CAD build for the part. Positions are in the model's coordinates, mm. Coordinates: 2 decimals unless noted, no trailing zeros. Loops run counter-clockwise (first coordinate to the right, second up) from the corner with the lowest first, then second, coordinate; pieces in that order, holes last.
1) Saw through at A-A, the plane x = 7. Write the cut outline in (y, z).
2) Pin check, flat tips, straight feed: pin 1 Ø8 at (x, y) = (11.5, -7) entering from +Z; pin 2 Ø5 at (x, z) = (2.5, 24.5) entering from +Y; pin 3 Ø4.5 at (x, z) = (7.5, 0) entering from -Y. Stop position of each tip, or through.
3) Saw through at B-B, the plane y = 0. Write the cut outline in (x, z), and give its area (3 significant figures).
4) Wall check: line 1 along X through (y, z) = (79, 0); line 2 along Z through (x, y) = (6, -70); line 3 along Y through (x, z) = (9.5, 43). Give the ranges that are in metal, low to high.
5) Two-plate mould, pull along Z, no slides. Class faces 1 (the flat face through (0, 17, 75)), 2 (the cylindrical face through (6, 81, 2)): +Z half, -Z half, draft (parallel to the pull), parting line (faces both ways), or undercut.
```python
from build123d import *

# Parameters (mm, degrees)
SKETCH1_W                      = 14
SKETCH1_H                      = 2
CUT_EXTRUDE1_REACH             = 123.723
SKETCH1_3_R                    = 2.5
CUT_EXTRUDE1_DIRECTION_2_REACH = 123.723
CUT_EXTRUDE2_REACH             = 123.697
CUT_EXTRUDE2_DIRECTION_2_REACH = 123.697


with BuildPart() as part:
    # Sketch1 → Revolve1 (revolve)
    with BuildSketch(Plane.XY, mode=Mode.PRIVATE) as revolve1_sk:
        with Locations((7, 77.5)):
            Rectangle(SKETCH1_W, SKETCH1_H)
        with BuildLine():
            ThreePointArc((0, 78.5), (7, 85.5), (14, 78.5))
            Line((14, 78.5), (0, 78.5))
        make_face()
    revolve(revolve1_sk.sketch.rotate(Axis((0, 0, 0), (1, 0, 0)), 180), axis=Axis((0, 0, 0), (1, 0, 0)))

    # Sketch1<3> → Cut-Extrude1 (cut, up to next)
    with BuildSketch(Plane.XY, mode=Mode.PRIVATE) as cut_extrude1_sk1:
        with Locations((7, 0)):
            Circle(SKETCH1_3_R)
    cut_extrude1_tool1 = extrude(cut_extrude1_sk1.sketch, amount=-CUT_EXTRUDE1_REACH, mode=Mode.PRIVATE) & part.part
    add(cut_extrude1_tool1.solids().sort_by_distance((7, 0, 0))[0], mode=Mode.SUBTRACT)

    # Sketch1<3> → Cut-Extrude1 direction 2 (cut, up to next)
    with BuildSketch(Plane.XY, mode=Mode.PRIVATE) as cut_extrude1_direction_2_sk1:
        with Locations((7, 0)):
            Circle(SKETCH1_3_R)
    cut_extrude1_direction_2_tool1 = extrude(cut_extrude1_direction_2_sk1.sketch, amount=CUT_EXTRUDE1_DIRECTION_2_REACH, mode=Mode.PRIVATE) & part.part
    add(cut_extrude1_direction_2_tool1.solids().sort_by_distance((7, 0, 0))[0], mode=Mode.SUBTRACT)

    # Sketch2 → Cut-Extrude2 (cut, up to next)
    with BuildSketch(Plane(origin=(0, 0, 0), x_dir=(1, 0, 0), z_dir=(0, 1, 0)), mode=Mode.PRIVATE) as cut_extrude2_sk1:
        with BuildLine():
            ThreePointArc((10, 0), (7.5, 2.5), (5, 0))
            Line((5, 0), (10, 0))
        make_face()
    cut_extrude2_tool1 = extrude(cut_extrude2_sk1.sketch, amount=-CUT_EXTRUDE2_REACH, mode=Mode.PRIVATE) & part.part
    # Sketch2 → Cut-Extrude2 (cut, up to next)
    with BuildSketch(Plane(origin=(0, 0, 0), x_dir=(1, 0, 0), z_dir=(0, 1, 0)), mode=Mode.PRIVATE) as cut_extrude2_sk2:
        with BuildLine():
            Line((10, 0), (5, 0))
            ThreePointArc((5, 0), (7.5, -2.5), (10, 0))
        make_face()
    cut_extrude2_tool2 = extrude(cut_extrude2_sk2.sketch, amount=-CUT_EXTRUDE2_REACH, mode=Mode.PRIVATE) & part.part
    # Sketch2 → Cut-Extrude2 (cut, up to next)
    with BuildSketch(Plane(origin=(0, 0, 0), x_dir=(1, 0, 0), z_dir=(0, 1, 0)), mode=Mode.PRIVATE) as cut_extrude2_sk3:
        with BuildLine():
            ThreePointArc((10, 0), (7.5, 2.5), (5, 0))
            Line((5, 0), (10, 0))
        make_face()
    cut_extrude2_tool3 = extrude(cut_extrude2_sk3.sketch, amount=-CUT_EXTRUDE2_REACH, mode=Mode.PRIVATE) & part.part
    # Sketch2 → Cut-Extrude2 (cut, up to next)
    with BuildSketch(Plane(origin=(0, 0, 0), x_dir=(1, 0, 0), z_dir=(0, 1, 0)), mode=Mode.PRIVATE) as cut_extrude2_sk4:
        with BuildLine():
            Line((10, 0), (5, 0))
            ThreePointArc((5, 0), (7.5, -2.5), (10, 0))
        make_face()
    cut_extrude2_tool4 = extrude(cut_extrude2_sk4.sketch, amount=-CUT_EXTRUDE2_REACH, mode=Mode.PRIVATE) & part.part
    add(cut_extrude2_tool1.solids().sort_by_distance((7.5, 0, -1.061033))[0], mode=Mode.SUBTRACT)
    add(cut_extrude2_tool2.solids().sort_by_distance((7.5, 0, 1.061033))[0], mode=Mode.SUBTRACT)
    add(cut_extrude2_tool3.solids().sort_by_distance((7.5, 0, -1.061033))[0], mode=Mode.SUBTRACT)
    add(cut_extrude2_tool4.solids().sort_by_distance((7.5, 0, 1.061033))[0], mode=Mode.SUBTRACT)

    # Sketch2 → Cut-Extrude2 direction 2 (cut, up to next)
    with BuildSketch(Plane(origin=(0, 0, 0), x_dir=(1, 0, 0), z_dir=(0, 1, 0)), mode=Mode.PRIVATE) as cut_extrude2_direction_2_sk1:
        with BuildLine():
            ThreePointArc((10, 0), (7.5, 2.5), (5, 0))
            Line((5, 0), (10, 0))
        make_face()
    cut_extrude2_direction_2_tool1 = extrude(cut_extrude2_direction_2_sk1.sketch, amount=CUT_EXTRUDE2_DIRECTION_2_REACH, mode=Mode.PRIVATE) & part.part
    # Sketch2 → Cut-Extrude2 direction 2 (cut, up to next)
    with BuildSketch(Plane(origin=(0, 0, 0), x_dir=(1, 0, 0), z_dir=(0, 1, 0)), mode=Mode.PRIVATE) as cut_extrude2_direction_2_sk2:
        with BuildLine():
            Line((10, 0), (5, 0))
            ThreePointArc((5, 0), (7.5, -2.5), (10, 0))
        make_face()
    cut_extrude2_direction_2_tool2 = extrude(cut_extrude2_direction_2_sk2.sketch, amount=CUT_EXTRUDE2_DIRECTION_2_REACH, mode=Mode.PRIVATE) & part.part
    # Sketch2 → Cut-Extrude2 direction 2 (cut, up to next)
    with BuildSketch(Plane(origin=(0, 0, 0), x_dir=(1, 0, 0), z_dir=(0, 1, 0)), mode=Mode.PRIVATE) as cut_extrude2_direction_2_sk3:
        with BuildLine():
            ThreePointArc((10, 0), (7.5, 2.5), (5, 0))
            Line((5, 0), (10, 0))
        make_face()
    cut_extrude2_direction_2_tool3 = extrude(cut_extrude2_direction_2_sk3.sketch, amount=CUT_EXTRUDE2_DIRECTION_2_REACH, mode=Mode.PRIVATE) & part.part
    # Sketch2 → Cut-Extrude2 direction 2 (cut, up to next)
    with BuildSketch(Plane(origin=(0, 0, 0), x_dir=(1, 0, 0), z_dir=(0, 1, 0)), mode=Mode.PRIVATE) as cut_extrude2_direction_2_sk4:
        with BuildLine():
            Line((10, 0), (5, 0))
            ThreePointArc((5, 0), (7.5, -2.5), (10, 0))
        make_face()
    cut_extrude2_direction_2_tool4 = extrude(cut_extrude2_direction_2_sk4.sketch, amount=CUT_EXTRUDE2_DIRECTION_2_REACH, mode=Mode.PRIVATE) & part.part
    add(cut_extrude2_direction_2_tool1.solids().sort_by_distance((7.5, 0, -1.061033))[0], mode=Mode.SUBTRACT)
    add(cut_extrude2_direction_2_tool2.solids().sort_by_distance((7.5, 0, 1.061033))[0], mode=Mode.SUBTRACT)
    add(cut_extrude2_direction_2_tool3.solids().sort_by_distance((7.5, 0, -1.061033))[0], mode=Mode.SUBTRACT)
    add(cut_extrude2_direction_2_tool4.solids().sort_by_distance((7.5, 0, 1.061033))[0], mode=Mode.SUBTRACT)


solid = part.part
```
Data:
1. outline: (-85.46, -2.45) arc R85.5 ccw to (-2.5, -85.46) - (-2.5, -76.46) arc R76.5 cw to (-76.46, -2.45) - close; (-85.46, 2.45) - (-76.46, 2.45) arc R76.5 cw to (-2.5, 76.46) - (-2.5, 85.46) arc R85.5 ccw to start; (2.5, -85.46) arc R85.5 ccw to (85.46, -2.45) - (76.46, -2.45) arc R76.5 cw to (2.5, -76.46) - close; (2.5, 76.46) arc R76.5 cw to (76.46, 2.45) - (85.46, 2.45) arc R85.5 ccw to (2.5, 85.46) - close
2. pin 1: stops at z = 85.28
2. pin 2: stops at y = 81.87
2. pin 3: passes through
3. outline: (0, -78.5) arc R7 ccw to (4.5, -85.04) - (4.5, -76.5) - (0, -76.5) - close; (0, 76.5) - (4.5, 76.5) - (4.5, 85.04) arc R7 ccw to (0, 78.5) - close; (9.5, -85.04) arc R7 ccw to (14, -78.5) - (14, -76.5) - (9.5, -76.5) - close; (9.5, 76.5) - (14, 76.5) - (14, 78.5) arc R7 ccw to (9.5, 85.04) - close
3. area: 121 mm2
4. line 1: x = 0.02 to 5, 10 to 13.98
4. line 2: z = -48.97 to -30.86, 30.86 to 48.97
4. line 3: y = -73.37 to -63.27, 63.27 to 73.37
5. face 1: draft
5. face 2: undercut
